Work out the finished part from the listing and answer in its coordinate system (mm). Round coordinates to 2 decimals unless told otherwise and drop trailing zeros. Order: outer loops, then holes, each group sorted by start corner. A loop starts at its lowest first (then second) coordinate and runs counter-clockwise, first axis right, second up. Notation, with made-up numbers: (35, -5.5) - (82, -5.5) arc R29 ccw to (82, 19.5) - close; hole circle Ø3 at (17.5, 17). An arc over 180 degrees is marked (long way). Put each result on its own line as item: value.
```python
from build123d import *

# Parameters (mm, degrees)
EXTRUDE_1_DEPTH     = 3
CUT_EXTRUDE_1_DEPTH = 3
SKETCH_3_R          = 5
CUT_EXTRUDE_2_DEPTH = 3
SKETCH_6_R          = 1
CUT_EXTRUDE_3_DEPTH = 3


with BuildPart() as part:
    # 草图1 → 凸台-拉伸1 (new body)
    with BuildSketch(Plane.XY):
        Polygon((11.895283312, 20.845067899), (-12.104716688, 20.724151483), (-24, -0.120916416), (-11.895283312, -20.845067899), (12.104716688, -20.724151483), (24, 0.120916416), align=None)
    extrude(amount=EXTRUDE_1_DEPTH)

    # 草图2 → 切除-拉伸1 (cut)
    with BuildSketch(Plane.XY.offset(3)):
        Polygon((10.250974371, 13.746627049), (9.387479018, 13.242270255), (12.514491143, 7.888599068), (13.377986495, 8.392955863), align=None)
        Polygon((13.018847937, 7.025103716), (13.88234329, 7.52946051), (17.009355414, 2.175789323), (16.145860061, 1.671432529), align=None)
        Polygon((6.779441055, -15.750917743), (6.774402935, -14.750930435), (0.574481622, -14.782166779), (0.579519742, -15.782154088), align=None)
        Polygon((-0.425505687, -14.787204899), (-0.420467566, -15.787192208), (-6.62038888, -15.818428552), (-6.625427, -14.818441244), align=None)
        Polygon((-17.030415426, 2.004290694), (-16.161881954, 1.50866018), (-13.088972765, 6.893567711), (-13.957506238, 7.389198225), align=None)
        Polygon((-12.59334225, 7.762101184), (-13.461875723, 8.257731698), (-10.388966534, 13.642639229), (-9.520433062, 13.147008715), align=None)
    extrude(amount=-CUT_EXTRUDE_1_DEPTH, mode=Mode.SUBTRACT)

    # 草图3 → 切除-拉伸2 (cut)
    with BuildSketch(Plane.XY.offset(3)):
        Circle(SKETCH_3_R)
    extrude(amount=-CUT_EXTRUDE_2_DEPTH, mode=Mode.SUBTRACT)

    # 草图6 → 切除-拉伸3 (cut)
    with BuildSketch(Plane.XY.offset(3)):
        with Locations((-0.100452801, 17.784593098)):
            Circle(SKETCH_6_R)
        with Locations((15.45213582, -8.805301872)):
            Circle(SKETCH_6_R)
        with Locations((-15.351683019, -8.979291227)):
            Circle(SKETCH_6_R)
    extrude(amount=-CUT_EXTRUDE_3_DEPTH, mode=Mode.SUBTRACT)


solid = part.part
```
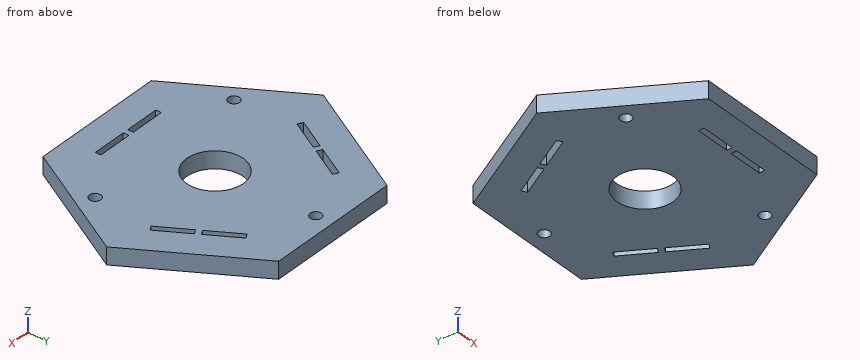
1) A cutting plane is placed at A-A on y = 12. Write down the section's boundary in (x, z).
Findings below:
outline: (-17.08, 0) - (-11.33, 0) - (-11.33, 3) - (-17.08, 3) - close; (-10.17, 0) - (10.11, 0) - (10.11, 3) - (-10.17, 3) - close; (11.27, 0) - (17.06, 0) - (17.06, 3) - (11.27, 3) - close
2) A cutting plane is placed at C-C on x = 19. Write down the section's boundary in (y, z).
Findings below:
outline: (-8.64, 0) - (8.68, 0) - (8.68, 3) - (-8.64, 3) - close
3) Straight lines are drawn through the part: L1, parallel to Y at x = 2, z = 0.55 (3 decimals); L2, parallel to Y at x = -1, z = 0.65; L3, parallel to X at y = 9.5, z = 2.8. For each, find the intervals that lie inside material, in ascending order. Write a range as from..to.
Findings below:
L1: y = -20.775..-15.775, -14.775..-4.583, 4.583..20.795
L2: y = -20.79..-15.79, -14.79..-4.9, 4.9..17.35, 18.22..20.78
L3: x = -18.51..-12.75, -11.6..11.57, 12.73..18.52
4) A cutting plane is placed at B-B on z = 1.35. Give the number of separate pieces and of enclosed holes in the cut face, then the cut area to 3 significant figures.
Findings below:
separate pieces: 1
enclosed holes: 10
area: 1,370 mm2
5) Given pin 1 Ø1.5 at (y, z) = (11, 1) entering from +X; pin 2 Ø1.5 at (y, z) = (2.5, 2) entering from -X, each flat-ended and moving along its own axis, determine where each tip first touches the part or whether it passes through.
Findings below:
pin 1: stops at x = 18.08
pin 2: stops at x = -22.93
